Read the model definition and answer for the solid it produces. Units are mm, in the model's axes. A direction names the side the tool comes from. Round coordinates to 2 decimals unless told otherwise and drop trailing zeros. Order: outer loops, then holes, each group sorted by start corner. A loop starts at its lowest first (then second) coordinate and runs counter-clockwise, first axis right, second up. Notation, with made-up numbers: (-9, 18.25) - (20, 18.25) arc R29 ccw to (20, 48.25) - close; hole circle Ø4 at (-3, 47). An arc over 180 degrees is marked (long way). One line per question, with ' | ' between items. Start each with the question number.
1) For faces 1 (the cylindrical face through (28.987, -16.013, -2.248)), 2 (the flat face through (25, -16, -3)), 3 (the flat face through (14, -1, 2)), 4 (the cylindrical face through (21.713, -15.887, 2.248)), determine the directions among +Z, -Z, +X, -X, +Y, -Y from which every point of the face is accessible in a straight line to the end or side of a thin tool.
2) Flat-ended cylindrical pins translate along their axes: pin 1 (8 mm diameter, centred on x = 22.5, y = -10, fed in from -Z); pin 2 (6 mm diameter, centred on x = 17.5, y = -7.5, fed in from -Z); pin 3 (5 mm diameter, centred on x = 16.5, z = 3.5, fed in from -Y); pin 4 (10 mm diameter, centred on x = 8, y = -4, fed in from -Z). Find the tip coordinate at first contact, or state that the pin passes through.
3) The part is cut by section A-A, the plane z = 0. Give the vertices of the cut face in (x, y), plus the area to 3 significant figures.
4) Straight lines are drawn through the part: line 1 (X direction, y = -4, z = -0.25); line 2 (Z direction, x = 2.75, y = 0.25); line 3 (X direction, y = 2.75, z = 3). For each, find the intervals that lie inside material, in ascending order. Write a range as from..to.
5) The part is cut by section B-B, the plane y = -14.5. Give the vertices of the cut face in (x, z).
6) The part is cut by section C-C, the plane x = 22.25. Give the vertices of the cut face in (y, z), plus the area to 3 significant figures.
7) The part is cut by section D-D, the plane x = 13.5. Give the vertices of the cut face in (y, z), plus the area to 3 significant figures.
from build123d import *

# Parameters (mm, degrees)
SKETCH1_R           = 3.5
BOSS_EXTRUDE1_DEPTH = 7
BOSS_EXTRUDE2_DEPTH = 8.7
FILLET1_R           = 2.5
FILLET2_R           = 1.5


with BuildPart() as part:
    # SurfaceCut1: read off the stored shape, not the designer's step
    # SurfaceCut1 outline → SurfaceCut1 (revolve)
    with BuildSketch(Plane.YX):
        with BuildLine():
            Line((0.5, 0), (1.434408923, 0.934408923))
            ThreePointArc((1.434408923, 0.934408923), (1.4807846, 1.007038752), (1.492296719, 1.092439376))
            Line((1.492296719, 1.092439376), (1.25, 4))
            Line((1.25, 4), (1.6, 4.4))
            Line((1.6, 4.4), (1.6, 5.5))
            Line((1.6, 5.5), (1.75, 5.65))
            Line((1.75, 5.65), (1.75, 14))
            Line((1.75, 14), (0, 14))
            Line((0, 14), (0, 0))
            Line((0, 0), (0.5, 0))
        make_face()
    revolve(axis=Axis((0, 0, 0), (1, 0, 0)))

    # Sketch1 → Boss-Extrude1 (add)
    with BuildSketch(Plane(origin=(14, 0, 0), x_dir=(0, 0, -1), z_dir=(1, 0, 0))):
        Circle(SKETCH1_R)
    extrude(amount=BOSS_EXTRUDE1_DEPTH)

    # Sketch2 → Boss-Extrude2 (add)
    with BuildSketch(Plane(origin=(21, 0, 0), x_dir=(0, 0, -1), z_dir=(1, 0, 0))):
        with BuildLine():
            Line((-4, -11.45), (-4.544657599, -0.220425293))
            ThreePointArc((-4.544657599, -0.220425293), (0, 4.55), (4.544657599, -0.220425293))
            Line((4.544657599, -0.220425293), (4, -11.45))
            Line((4, -11.45), (3, -11.45))
            Line((3, -11.45), (3, -20.45))
            Line((3, -20.45), (-3, -20.45))
            Line((-3, -20.45), (-3, -11.45))
            Line((-3, -11.45), (-4, -11.45))
        make_face()
    extrude(amount=BOSS_EXTRUDE2_DEPTH)

    # Fillet1
    fillet1_edges = [part.edges().sort_by_distance(p)[0] for p in [
        (21, -15.95, 3),
        (21, -15.95, -3),
        (29.7, -15.95, 3),
        (29.7, -15.95, -3),
    ]]
    fillet(fillet1_edges, radius=FILLET1_R)

    # Fillet2
    fillet2_edges = [part.edges().sort_by_distance(p)[0] for p in [
        (29.7, 4.55, 0),
        (29.7, -5.835212647, 4.272328799),
        (29.7, -5.835212647, -4.272328799),
    ]]
    fillet(fillet2_edges, radius=FILLET2_R)


solid = part.part
Values:
1) face 1: -Z, +X, -Y | face 2: -Z, +X, -X, -Y | face 3: -X | face 4: +Z, -X, -Y
2) pin 1: stops at z = -4.26 | pin 2: passes through | pin 3: stops at y = -3.35 | pin 4: stops at z = -1.75
3) outline: (0, -0.5) - (0.93, -1.43) arc R0.2 ccw to (1.09, -1.49) - (4, -1.25) - (4.4, -1.6) - (5.5, -1.6) - (5.65, -1.75) - (14, -1.75) - (14, -3.5) - (21, -3.5) - (21, -20.45) - (29.7, -20.45) - (29.7, 3.05) arc R1.5 ccw to (28.2, 4.55) - (21, 4.55) - (21, 3.5) - (14, 3.5) - (14, 1.75) - (5.65, 1.75) - (5.5, 1.6) - (4.4, 1.6) - (4, 1.25) - (1.09, 1.49) arc R0.2 ccw to (0.93, 1.43) - (0, 0.5) - close | area: 311 mm^2
4) line 1: x = 21..29.7 | line 2: z = -1.33..1.33 | line 3: x = 21..29.3
5) outline: (21, -0.5) arc R2.5 ccw to (23.5, -3) - (27.2, -3) arc R2.5 ccw to (29.7, -0.5) - (29.7, 0.5) arc R2.5 ccw to (27.2, 3) - (23.5, 3) arc R2.5 ccw to (21, 0.5) - close
6) outline: (-20.45, -2.67) - (-11.45, -2.67) - (-11.45, -4) - (-0.22, -4.54) arc R4.55 ccw (long way) to (-0.22, 4.54) - (-11.45, 4) - (-11.45, 2.67) - (-20.45, 2.67) - close | area: 178 mm^2
7) outline: circle Ø3.5 at (0, 0) | area: 9.62 mm^2
